from build123d import *

# Parameters (mm, degrees)
CYLINDER002_R     = 2
CYLINDER002_DEPTH = 10
CYLINDER003_R     = 2
CYLINDER003_DEPTH = 10
BOX004_W          = 2
BOX004_H          = 30
BOX004_DEPTH      = 20
FILLET004_R       = 3
FILLET005_R       = 1.9
CYLINDER_R        = 2
CYLINDER_DEPTH    = 10
CYLINDER001_R     = 2
CYLINDER001_DEPTH = 10
BOX003_W          = 2
BOX003_H          = 30
BOX003_DEPTH      = 20
FILLET003_R       = 3
FILLET006_R       = 1.9
BOX002_W          = 30
BOX002_H          = 40
BOX002_DEPTH      = 10
FILLET002_R       = 3
BOX001_W          = 30
BOX001_H          = 20
BOX001_DEPTH      = 10
FILLET001_R       = 3
BOX_W             = 50
BOX_H             = 100
BOX_DEPTH         = 2
FILLET_R          = 2


with BuildPart() as cilindre002:
    # Cylinder002 → Cylinder002 (new body)
    with BuildSketch(Plane(origin=(-4, 7, 11), x_dir=(0, 0, -1), z_dir=(1, 0, 0))):
        Circle(CYLINDER002_R)
    extrude(amount=CYLINDER002_DEPTH)


with BuildPart() as cilindre003:
    # Cylinder003 → Cylinder003 (new body)
    with BuildSketch(Plane(origin=(-4, 23, 11), x_dir=(0, 0, -1), z_dir=(1, 0, 0))):
        Circle(CYLINDER003_R)
    extrude(amount=CYLINDER003_DEPTH)


with BuildPart() as fillet005:
    # Box004 → Box004 (new body)
    with BuildSketch(Plane.XY):
        with Locations((1, 15)):
            Rectangle(BOX004_W, BOX004_H)
    extrude(amount=BOX004_DEPTH)

    # Fillet004
    fillet004_edges = [fillet005.edges().sort_by_distance(p)[0] for p in [
        (1, 0, 20),
        (1, 30, 20),
    ]]
    fillet(fillet004_edges, radius=FILLET004_R)

    # Cut004: cut Cilindre003
    add(cilindre003.part, mode=Mode.SUBTRACT)

    # Cut005: cut Cilindre002
    add(cilindre002.part, mode=Mode.SUBTRACT)


with BuildPart() as fillet005_1:
    # Cut005 placement: moved
    add(fillet005.part.moved(Location((52, 0, 0))))

    # Fillet005
    fillet005_edges = [fillet005_1.edges().sort_by_distance(p)[0] for p in [
        (54, 15, 0),
    ]]
    fillet(fillet005_edges, radius=FILLET005_R)


with BuildPart() as cilindre:
    # Cylinder → Cylinder (new body)
    with BuildSketch(Plane(origin=(-4, 7, 11), x_dir=(0, 0, -1), z_dir=(1, 0, 0))):
        Circle(CYLINDER_R)
    extrude(amount=CYLINDER_DEPTH)


with BuildPart() as cilindre001:
    # Cylinder001 → Cylinder001 (new body)
    with BuildSketch(Plane(origin=(-4, 23, 11), x_dir=(0, 0, -1), z_dir=(1, 0, 0))):
        Circle(CYLINDER001_R)
    extrude(amount=CYLINDER001_DEPTH)


with BuildPart() as fillet006:
    # Box003 → Box003 (new body)
    with BuildSketch(Plane.XY):
        with Locations((1, 15)):
            Rectangle(BOX003_W, BOX003_H)
    extrude(amount=BOX003_DEPTH)

    # Fillet003
    fillet003_edges = [fillet006.edges().sort_by_distance(p)[0] for p in [
        (1, 0, 20),
        (1, 30, 20),
    ]]
    fillet(fillet003_edges, radius=FILLET003_R)

    # Cut002: cut Cilindre001
    add(cilindre001.part, mode=Mode.SUBTRACT)

    # Cut003: cut Cilindre
    add(cilindre.part, mode=Mode.SUBTRACT)

    # Fillet006
    fillet006_edges = [fillet006.edges().sort_by_distance(p)[0] for p in [
        (0, 15, 0),
    ]]
    fillet(fillet006_edges, radius=FILLET006_R)


with BuildPart() as fusion:
    # Fusion base: copy of Fillet006
    add(fillet006.part)

    # Fusion: union Fillet005
    add(fillet005_1.part)


with BuildPart() as forat2:
    # Box002 → Box002 (new body)
    with BuildSketch(Plane.XY):
        with Locations((15, 20)):
            Rectangle(BOX002_W, BOX002_H)
    extrude(amount=BOX002_DEPTH)

    # Fillet002
    fillet002_edges = [forat2.edges().sort_by_distance(p)[0] for p in [
        (0, 0, 5),
        (0, 40, 5),
        (30, 0, 5),
        (30, 40, 5),
    ]]
    fillet(fillet002_edges, radius=FILLET002_R)


with BuildPart() as forat2_1:
    # Fillet002 placement: moved
    add(forat2.part.moved(Location((10, 10, -5))))


with BuildPart() as forat1:
    # Box001 → Box001 (new body)
    with BuildSketch(Plane.XY):
        with Locations((15, 10)):
            Rectangle(BOX001_W, BOX001_H)
    extrude(amount=BOX001_DEPTH)

    # Fillet001
    fillet001_edges = [forat1.edges().sort_by_distance(p)[0] for p in [
        (0, 0, 5),
        (0, 20, 5),
        (30, 0, 5),
        (30, 20, 5),
    ]]
    fillet(fillet001_edges, radius=FILLET001_R)


with BuildPart() as forat1_1:
    # Fillet001 placement: moved
    add(forat1.part.moved(Location((10, 70, -5))))


with BuildPart() as base:
    # Box → Box (new body)
    with BuildSketch(Plane.XY):
        with Locations((25, 50)):
            Rectangle(BOX_W, BOX_H)
    extrude(amount=BOX_DEPTH)

    # Fillet
    fillet_edges = [base.edges().sort_by_distance(p)[0] for p in [
        (0, 100, 1),
        (50, 100, 1),
    ]]
    fillet(fillet_edges, radius=FILLET_R)

    # Cut: cut forat1
    add(forat1_1.part, mode=Mode.SUBTRACT)

    # Cut001: cut forat2
    add(forat2_1.part, mode=Mode.SUBTRACT)


with BuildPart() as base_1:
    # Cut001 placement: moved
    add(base.part.moved(Location((2, 0, 0))))


with BuildPart() as fusion001:
    # Fusion001 base: copy of Fillet006
    add(fillet006.part)

    # Fusion001: union Fillet005, Fusion, base
    add(fillet005_1.part)
    add(fusion.part)
    add(base_1.part)


solid = fusion001.part
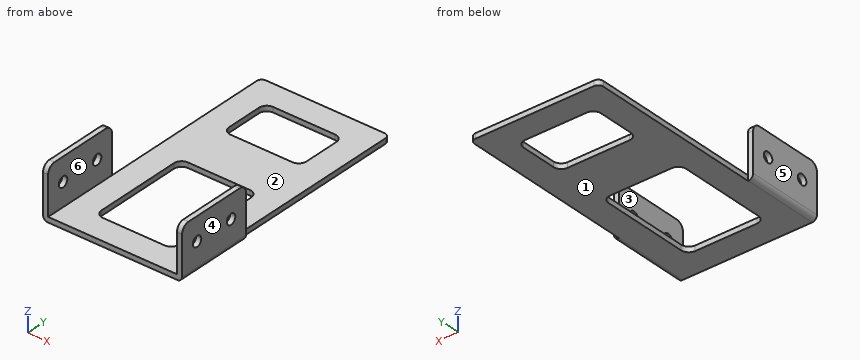
The listing builds one solid part. Answer for the finished solid, in the listing's coordinates (mm). Face numbers are marked on the shaded views. A direction names the side the tool comes from. Give positions to 0.01 mm unless a question says otherwise; leave off trailing zeros. Order: outer loops, then holes, each group sorted by start corner. A loop starts at its lowest first (then second) coordinate and runs counter-clockwise, first axis right, second up. Notation, with made-up numbers: (-16, 21.25) - (31, 21.25) arc R19 ccw to (31, 42.25) - close; hole circle Ø6 at (61, 57). An arc over 180 degrees is marked (long way). One line per item, written item: value. Start each with the question number.
1) A cutting plane is placed at B-B on x = 37.5. Give the vertices of the cut face in (y, z).
2) The mould has two halves that part along X. Classify the marked faces 1, 2, 3 and 4: released by +X, released by -X, zero draft, split by the parting line, or undercut.
3) A cutting plane is placed at D-D on y = 23. Give the vertices of the cut face in (x, z), then the cut area to 3 significant figures.
4) A cutting plane is placed at A-A on z = 11. Give the vertices of the cut face in (x, y), then the cut area to 3 significant figures.
5) A cutting plane is placed at C-C on y = 45.5. Give the vertices of the cut face in (x, z), then the cut area to 3 significant figures.
6) Given pin 1 Ø10 at (x, y) = (9, 24) entering from +Z; pin 2 Ø1.6 at (x, z) = (53.5, 5.5) entering from +Y; pin 3 Ø10 at (y, z) = (49.5, 8) entering from -X; pin 4 Ø12 at (y, z) = (78.5, 2.5) entering from -X, each flat-ended and moving along its own axis, determine where each tip first touches the part or whether it passes through.
7) A tool of negligible diameter and unlimited length cuts with its end or side. For the marked faces 5 and 6, from which of +Z, -Z, +X, -X, +Y, -Y can it reach the whole face along a straight path? Write none if from no direction.
8) Find the intervals of material crossed by L1, parallel to Y at x = 53.5, z = 11; L2, parallel to X at y = 12.5, z = 13.75; L3, parallel to Z at x = 50, y = 46, in increasing order.
Answer sheet:
1. outline: (0, 0) - (10, 0) - (10, 2) - (0, 2) - close; (50, 0) - (70, 0) - (70, 2) - (50, 2) - close; (90, 0) - (100, 0) - (100, 2) - (90, 2) - close
2. face 1: zero draft
2. face 2: undercut
2. face 3: undercut
2. face 4: released by +X
3. outline: (0, 1.9) arc R1.9 ccw to (1.9, 0) - (12, 0) - (12, 2) - (2, 2) - (2, 9) - (0, 9) - close; (0, 13) - (2, 13) - (2, 20) - (0, 20) - close; (42, 0) - (52.1, 0) arc R1.9 ccw to (54, 1.9) - (54, 9) - (52, 9) - (52, 2) - (42, 2) - close; (52, 13) - (54, 13) - (54, 20) - (52, 20) - close
3. area: 102 mm2
4. outline: (0, 0) - (2, 0) - (2, 5) - (0, 5) - close; (0, 9) - (2, 9) - (2, 21) - (0, 21) - close; (0, 25) - (2, 25) - (2, 30) - (0, 30) - close; (52, 0) - (54, 0) - (54, 5) - (52, 5) - close; (52, 9) - (54, 9) - (54, 21) - (52, 21) - close; (52, 25) - (54, 25) - (54, 30) - (52, 30) - close
4. area: 88.0 mm2
5. outline: (2, 0) - (12, 0) - (12, 2) - (2, 2) - close; (42, 0) - (52, 0) - (52, 2) - (42, 2) - close
5. area: 40.0 mm2
6. pin 1: stops at z = 2
6. pin 2: stops at y = 30
6. pin 3: passes through
6. pin 4: stops at x = 2
7. face 5: +Z, -Z, -X, +Y, -Y
7. face 6: +Z, +Y, -Y
8. L1: y = 0 to 5, 9 to 21, 25 to 30
8. L2: x = 0 to 2, 52 to 54
8. L3: z = 0 to 2
